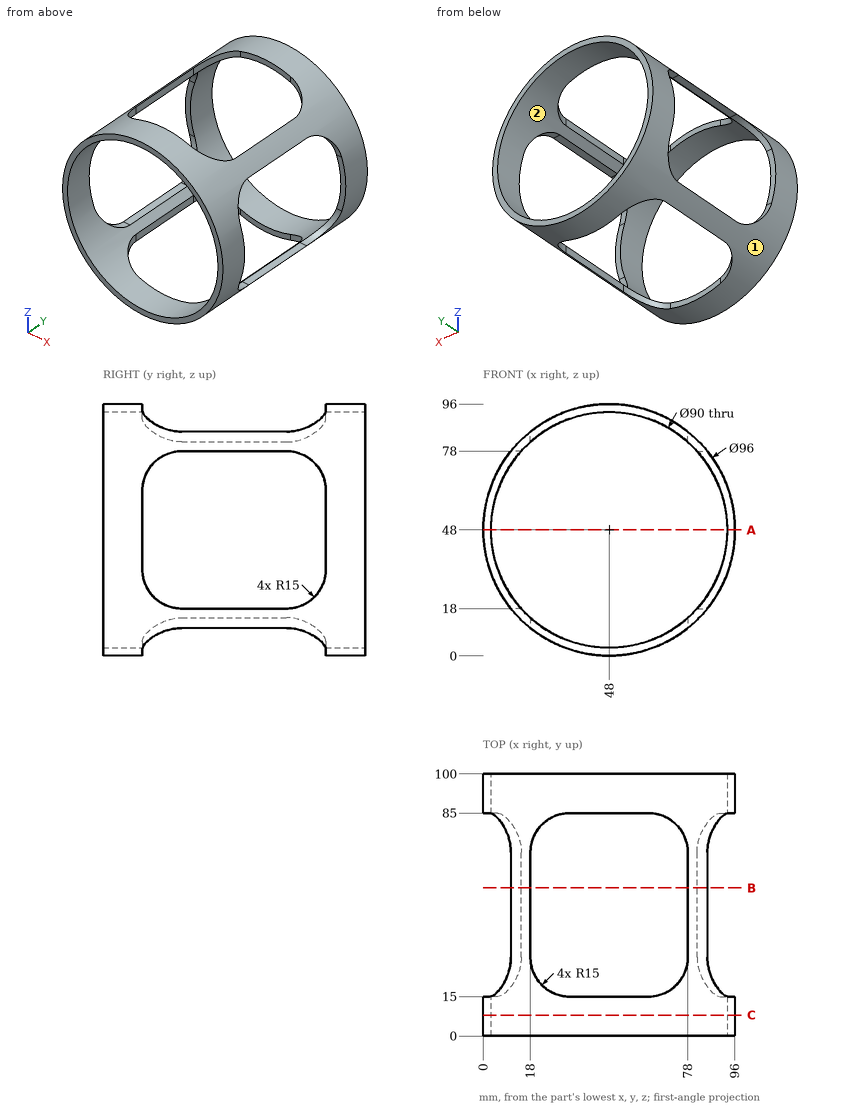
Source: three-view drawing plus pictorial views. Frame: mm from the lowest corner of the part. Coordinates: 2 decimals unless noted, no trailing zeros. Order: outer loops, then holes, each group sorted by start corner. A loop starts at its lowest first (then second) coordinate and runs counter-clockwise, first axis right, second up. Notation, with made-up numbers: M -27,29 L 23,29 A12 ccw 23,39 Z; hole C 22.25,-31.75 d9. An arc over 180 degrees is marked long. Answer in a Markdown table with one row per item.
(1) Section query C-C, the plane y = 8. Output: boundary loops of the cut face in (x, z).
Numbers:
| item | result |
|---|---|
| outline | C 48,48 d96; hole C 48,48 d90 |
(2) Draft query along Z for the marked faces 1 and 2. Return one class per face: pulls with the +Z half, pulls with the -Z half, needs draft (parallel to the pull), parting line crosses it, or undercut.
Numbers:
| item | result |
|---|---|
| face 1 | parting line crosses it |
| face 2 | undercut |
(3) Section query B-B, the plane y = 56.5. Output: boundary loops of the cut face in (x, z).
Numbers:
| item | result |
|---|---|
| outline | M 10.53,18 A48 ccw 18,10.53 L 18,14.46 A45 cw 14.46,18 Z; M 10.53,78 L 14.46,78 A45 cw 18,81.54 L 18,85.47 A48 ccw Z; M 78,10.53 A48 ccw 85.47,18 L 81.54,18 A45 cw 78,14.46 Z; M 78,81.54 A45 cw 81.54,78 L 85.47,78 A48 ccw 78,85.47 Z |
(4) Section query A-A, the plane z = 48. Output: boundary loops of the cut face in (x, y).
Numbers:
| item | result |
|---|---|
| outline | M 0,0 L 3,0 L 3,15 L 0,15 Z; M 0,85 L 3,85 L 3,100 L 0,100 Z; M 93,0 L 96,0 L 96,15 L 93,15 Z; M 93,85 L 96,85 L 96,100 L 93,100 Z |
(5) Material intervals for line 1 (X direction, y = 15, z = 78); line 2 (X direction, y = 6, z = 29); line 3 (Z direction, x = 45, y = 94), sorted ascending. Write a range as [from, to].
Numbers:
| item | result |
|---|---|
| line 1 | x = [10.53, 14.46], [81.54, 85.47] |
| line 2 | x = [3.92, 7.21], [88.79, 92.08] |
| line 3 | z = [0.09, 3.1], [92.9, 95.91] |
(6) Contact query for flat-ended pins moving along their axis: pin 1 Ø4.5 at (y, z) = (48, 13) entering from -X; pin 2 Ø4 at (x, y) = (78.5, 42.5) entering from -Z; pin 3 Ø4.5 at (x, y) = (82.5, 60) entering from -Z; pin 4 Ø6 at (x, z) = (3.5, 52) entering from +Y. Output: stop coordinate, or through.
Numbers:
| item | result |
|---|---|
| pin 1 | stops at x = 12.91 |
| pin 2 | stops at z = 10.53 |
| pin 3 | stops at z = 12.45 |
| pin 4 | stops at y = 100 |
